Design review of the part built by this model. Coordinates are the model's own, in mm. Face numbers are marked on the shaded views. A direction names the side the tool comes from. Coordinates: 2 decimals unless noted, no trailing zeros. Write each loop counter-clockwise with the first axis right and the second up, starting at its lowest first coordinate (ties: lowest second). Pieces come first, ordered by that corner, then holes. Notation, with made-up numbers: (30, 15.5) - (87, 15.5) arc R17 ccw to (87, 38.5) - close; hole circle Ø4 at (26.5, 20). An arc over 180 degrees is marked (long way). One line per item, written item: value.
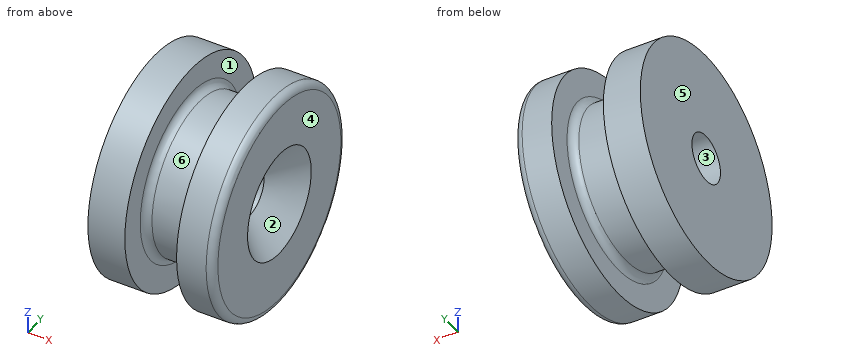
from build123d import *

# Parameters (mm, degrees)
FILLET1_R     = 1
FILLET2_R     = 1
CHAMFER1_SIZE = 4


with BuildPart() as part:
    # Sketch1 → Revolve1 (revolve)
    with BuildSketch(Plane.XY, mode=Mode.PRIVATE) as revolve1_sk:
        Polygon((12, 15), (17, 15), (17, 3.25), (0, 3.25), (0, 15), (5, 15), (5, 10.5), (12, 10.5), align=None)
    revolve(revolve1_sk.sketch.rotate(Axis((-8.121930128, 0, 0), (1, 0, 0)), 90), axis=Axis((-8.121930128, 0, 0), (1, 0, 0)))

    # Fillet1
    fillet1_edges = [part.edges().sort_by_distance(p)[0] for p in [
        (17, 0, -15),
    ]]
    fillet(fillet1_edges, radius=FILLET1_R)

    # Fillet2
    fillet2_edges = [part.edges().sort_by_distance(p)[0] for p in [
        (12, 0, -10.5),
        (5, 0, -10.5),
    ]]
    fillet(fillet2_edges, radius=FILLET2_R)

    # Chamfer1
    chamfer1_edges = [part.edges().sort_by_distance(p)[0] for p in [
        (17, 0, -3.25),
    ]]
    chamfer(chamfer1_edges, length=CHAMFER1_SIZE)


solid = part.part
1. Wall thickness on line 1 along X through (y, z) = (-11, -3); line 2 along Y through (x, z) = (6.75, 0); line 3 along Z through (x, y) = (13.75, 2): over which ranges is each line inside the solid? List them lowest first.
Answer block:
line 1: x = 0 to 5, 12 to 17
line 2: y = -10.5 to -3.25, 3.25 to 10.5
line 3: z = -14.87 to -3.46, 3.46 to 14.87
2. Mouldability with a two-part tool opening along X and no side actions: class the marked faces 3, 4, 5 and 6 as released by +X, released by -X, zero draft, split by the parting line, or undercut.
Answer block:
face 3: zero draft
face 4: released by +X
face 5: released by -X
face 6: undercut
3. Consider section C-C, the plane x = 7.75. Write out the cut boundary in (y, z).
Answer block:
outline: circle Ø21 at (0, 0); hole circle Ø6.5 at (0, 0)
4. Insertion check: pin 1 Ø5 at (x, z) = (15, -4) entering from -Y; pin 2 Ø15 at (y, z) = (-4, 4.5) entering from -X; pin 3 Ø1.5 at (y, z) = (1, 5) entering from +X; pin 4 Ø8 at (x, y) = (15, -11.5) entering from +Z. Each pin has a flat end and moves straight along its axis. Give the tip position at first contact, or say it passes through.
Answer block:
pin 1: stops at y = -14.92
pin 2: stops at x = 0
pin 3: stops at x = 15.6
pin 4: stops at z = 12.99
5. For the marked faces 1 and 2, list the 3-axis set-ups (+Z, -Z, +X, -X, +Y, -Y) from which the entire face can be reached by the end or side of a thin tool; tool diameter is ignored.
Answer block:
face 1: none
face 2: +X
6. Consider section D-D, the plane x = 2. Write out the cut boundary in (y, z), then the cut area to 3 significant figures.
Answer block:
outline: circle Ø30 at (0, 0); hole circle Ø6.5 at (0, 0)
area: 674 mm^2
7. Consider section A-A, the plane y = 0. Write out the cut boundary in (x, z), then the cut area to 3 significant figures.
Answer block:
outline: (0, -15) - (5, -15) - (5, -11.5) arc R1 cw to (6, -10.5) - (11, -10.5) arc R1 cw to (12, -11.5) - (12, -15) - (16, -15) arc R1 ccw to (17, -14) - (17, -7.25) - (13, -3.25) - (0, -3.25) - close; (0, 3.25) - (13, 3.25) - (17, 7.25) - (17, 14) arc R1 ccw to (16, 15) - (12, 15) - (12, 11.5) arc R1 cw to (11, 10.5) - (6, 10.5) arc R1 cw to (5, 11.5) - (5, 15) - (0, 15) - close
area: 321 mm^2
